from build123d import *

# Parameters (mm, degrees)
CROQUIS1_R                   = 7
SALIENTE_EXTRUIR1_DEPTH      = 10
CROQUIS1_3_R                 = 13
CROQUIS1_3_R_2               = 7
SALIENTE_EXTRUIR2_DEPTH      = 2
TALADRO_DE_MARGEN_PARA_M31_D = 3.4
CHAFL_N1_SIZE                = 1
REDONDEO2_R                  = 1
CHAFL_N2_SIZE                = 1


with BuildPart() as part:
    # Croquis1 → Saliente-Extruir1 (new body)
    # profile 1 of 5: a face of its own
    with BuildSketch(Plane.XY):
        Circle(CROQUIS1_R)
        with BuildLine():
            Line((-1.5, 5), (0, 5))
            Line((0, 5), (1.5, 5))
            Line((1.5, 5), (1.5, 4.769696007))
            ThreePointArc((1.5, 4.769696007), (4.031128874, 2.958039892), (5, 0))
            ThreePointArc((5, 0), (-2.958039892, -4.031128874), (-1.5, 4.769696007))
            Line((-1.5, 4.769696007), (-1.5, 5))
        make_face(mode=Mode.SUBTRACT)
    # profile 2 of 5: a face of its own
    with BuildSketch(Plane.XY):
        with BuildLine():
            Line((0, 5), (0, 2))
            Line((0, 2), (1.5, 2))
            Line((1.5, 2), (1.5, 4.769696007))
            ThreePointArc((1.5, 4.769696007), (0.758788496, 4.942088629), (0, 5))
        make_face()
    # profile 3 of 5: a face of its own
    with BuildSketch(Plane.XY):
        with BuildLine():
            Line((-1.5, 2), (0, 2))
            Line((0, 2), (0, 5))
            ThreePointArc((0, 5), (-0.758788496, 4.942088629), (-1.5, 4.769696007))
            Line((-1.5, 4.769696007), (-1.5, 2))
        make_face()
    # profile 4 of 5: a face of its own
    with BuildSketch(Plane.XY):
        with BuildLine():
            Line((1.5, 5), (0, 5))
            ThreePointArc((0, 5), (0.758788496, 4.942088629), (1.5, 4.769696007))
            Line((1.5, 4.769696007), (1.5, 5))
        make_face()
    # profile 5 of 5: a face of its own
    with BuildSketch(Plane.XY):
        with BuildLine():
            ThreePointArc((-1.5, 4.769696007), (-0.758788496, 4.942088629), (0, 5))
            Line((0, 5), (-1.5, 5))
            Line((-1.5, 5), (-1.5, 4.769696007))
        make_face()
    extrude(amount=-SALIENTE_EXTRUIR1_DEPTH)

    # Croquis1<3> → Saliente-Extruir2 (add)
    with BuildSketch(Plane.XY):
        Circle(CROQUIS1_3_R)
        Circle(CROQUIS1_3_R_2, mode=Mode.SUBTRACT)
    extrude(amount=-SALIENTE_EXTRUIR2_DEPTH)

    # Taladro de margen para M31 (through all)
    with Locations(Plane.XY):
        with Locations((0, 10.5), (10.5, 0), (0, -10.5), (-10.5, 0), (0, 0)):
            Hole(TALADRO_DE_MARGEN_PARA_M31_D / 2)

    # Chaflán1
    chafl_n1_edges = [part.edges().sort_by_distance(p)[0] for p in [
        (-1.5, 3.384848004, -10),
        (0, 2, -10),
        (1.5, 3.384848004, -10),
        (0, -5, -10),
    ]]
    chamfer(chafl_n1_edges, length=CHAFL_N1_SIZE)

    # Redondeo2
    # the kernel refuses this fillet: 1 mm, written as the material it adds along each edge
    with BuildSketch(Plane(origin=(0, 0, -2), x_dir=(1, 0, 0), z_dir=(0, -1, 0))) as redondeo2_piece_1:
        with BuildLine():
            CenterArc((7 + REDONDEO2_R, -REDONDEO2_R), REDONDEO2_R, 90, 90)
            Line((7 + REDONDEO2_R, 0), (7, 0))
            Line((7, 0), (7, -REDONDEO2_R))
        make_face()
    revolve(axis=Axis((0, 0, -2), (0, 0, 1)))
    # the kernel refuses this fillet: 1 mm, written as the material it takes off along each edge
    with BuildSketch(Plane(origin=(0, 0, -2), x_dir=(1, 0, 0), z_dir=(0, -1, 0))) as redondeo2_2_piece_1:
        with BuildLine():
            CenterArc((13 - REDONDEO2_R, REDONDEO2_R), REDONDEO2_R, 270, 90)
            Line((13, REDONDEO2_R), (13, 0))
            Line((13, 0), (13 - REDONDEO2_R, 0))
        make_face()
    revolve(axis=Axis((0, 0, -2), (0, 0, 1)), mode=Mode.SUBTRACT)
    with BuildSketch(Plane(origin=(0, 0, -10), x_dir=(1, 0, 0), z_dir=(0, -1, 0))) as redondeo2_2_piece_2:
        with BuildLine():
            CenterArc((7 - REDONDEO2_R, REDONDEO2_R), REDONDEO2_R, 270, 90)
            Line((7, REDONDEO2_R), (7, 0))
            Line((7, 0), (7 - REDONDEO2_R, 0))
        make_face()
    revolve(axis=Axis((0, 0, -10), (0, 0, 1)), mode=Mode.SUBTRACT)

    # Chaflán2
    chafl_n2_edges = [part.edges().sort_by_distance(p)[0] for p in [
        (1.5, 3.384848004, 0),
        (0, 2, 0),
        (-1.5, 3.384848004, 0),
        (0, -5, 0),
    ]]
    chamfer(chafl_n2_edges, length=CHAFL_N2_SIZE)


solid = part.part
Check sheet for the modelled part. Datum: model origin and axes. Units: mm. A direction names the side the tool comes from. Round coordinates to 2 decimals unless told otherwise and drop trailing zeros. Order: outer loops, then holes, each group sorted by start corner. A loop starts at its lowest first (then second) coordinate and runs counter-clockwise, first axis right, second up.
(1) Draft check along X on faces 1 (the cylindrical face through (-10.316, -7.91, -0.493)), 2 (the flat face through (-1.5, 3, -5)), 3 (the flat face through (-1, 4, -0.5)), 4 (the flat face through (6, -3, 0)). Enter one of: pulls with the +X half, pulls with the -X half, needs draft (parallel to the pull), parting line crosses it, or undercut.
(2) Cross-section at B-B, the plane x = 0. Enter the section's corners in (y, z), and give its area (3 significant figures).
(3) Go/stop test with flat-tipped pins: P1, Ø1.5, axis at x = 2, z = -8, coming from the -Y side; P2, Ø6, axis at y = -1.5, z = -5.5, coming from the +X side; P3, Ø3.5, axis at x = -0.5, z = -5.5, coming from the -Y side. Record where each tip stops, or that it passes through.
(4) Access from +Z, -Z, +X, -X, +Y, -Y to the whole of each face (thin tool, end or side, straight path). Record for faces 5 (the flat face through (0, 5, -10)), 6 (the flat face through (-1, 4, -9.5)), 7 (the flat face through (0, 2, -5)), 8 (the flat face through (1, 4, -0.5)).
(5) Scan lines: probe 1 along Y at (x, z) = (0, -5); probe 2 along Y at (x, z) = (0, -0.6); probe 3 along X at (y, z) = (-0.25, -5.5). Record each from-to range of solid material in increasing order.
(6) Cross-section at A-A, the plane z = -4.75. Enter the section's corners in (x, y).
Check sheet entries:
1. face 1: parting line crosses it
1. face 2: undercut
1. face 3: undercut
1. face 4: needs draft
2. outline: (-13, -1) arc R1 ccw to (-12.2, -1.98) - (-12.2, 0) - (-13, 0) - close; (-8.8, -2) - (-8, -2) arc R1 cw to (-7, -3) - (-7, -9) arc R1 ccw to (-6, -10) - (-5, -9) - (-5, -1) - (-6, 0) - (-8.8, 0) - close; (2, -9) - (3, -10) - (6, -10) arc R1 ccw to (7, -9) - (7, -3) arc R1 cw to (8, -2) - (8.8, -2) - (8.8, 0) - (3, 0) - (2, -1) - close; (12.2, -1.98) arc R1 ccw to (13, -1) - (13, 0) - (12.2, 0) - close
2. area: 78.0 mm2
3. P1: stops at y = -6.89
3. P2: stops at x = 7.05
3. P3: stops at y = -7
4. face 5: -Z, +X, -X, +Y, -Y
4. face 6: -Z
4. face 7: +Z, -Z
4. face 8: +Z
5. probe 1: y = -7 to -5, 2 to 7
5. probe 2: y = -13 to -12.2, -8.8 to -5.4, 2.4 to 8.8, 12.2 to 13
5. probe 3: x = -7 to -4.99, 4.99 to 7
6. outline: circle Ø14 at (0, 0); hole (-1.5, 2) - (-1.5, 4.77) arc R5 ccw (long way) to (1.5, 4.77) - (1.5, 2) - close
